Source: CAD feature listing. Evaluate the final solid. Frame: model axes, mm. Give positions to 0.01 mm unless a question says otherwise; leave off trailing zeros. Order: outer loops, then holes, each group sorted by start corner. A loop starts at its lowest first (then second) coordinate and runs counter-clockwise, first axis right, second up. Notation, with made-up numbers: (-8.5, 55.25) - (9.5, 55.25) arc R18 cw to (9.5, 78.25) - close; hole circle Ø7 at (66.5, -14). An arc over 180 degrees is marked (long way). Answer as CSV lines item,"result".
```python
from build123d import *

# Parameters (mm, degrees)
SKETCH1_W           = 62
SKETCH1_H           = 35
BOSS_EXTRUDE1_DEPTH = 5
SKETCH2_R           = 2.5
CUT_EXTRUDE1_DEPTH  = 6
SKETCH3_R           = 2.5
SKETCH3_R_2         = 5
CUT_EXTRUDE2_DEPTH  = 6


with BuildPart() as part:
    # Sketch1 → Boss-Extrude1 (new body)
    with BuildSketch(Plane(origin=(0, 0, 0), x_dir=(1, 0, 0), z_dir=(0, 1, 0))):
        with Locations((31, 17.5)):
            Rectangle(SKETCH1_W, SKETCH1_H)
    extrude(amount=BOSS_EXTRUDE1_DEPTH)

    # Sketch2 → Cut-Extrude1 (cut, through all)
    with BuildSketch(Plane(origin=(0, 5, 0), x_dir=(1, 0, 0), z_dir=(0, 1, 0))):
        with Locations((5, 30)):
            Circle(SKETCH2_R)
        with Locations((5, 5)):
            Circle(SKETCH2_R)
    extrude(amount=-CUT_EXTRUDE1_DEPTH, mode=Mode.SUBTRACT)

    # Sketch3 → Cut-Extrude2 (cut, through all)
    with BuildSketch(Plane(origin=(0, 5, 0), x_dir=(1, 0, 0), z_dir=(0, 1, 0))):
        with Locations((56, 29)):
            Circle(SKETCH3_R)
        with Locations((56, 6)):
            Circle(SKETCH3_R)
        with Locations((33, 28.877597721)):
            Circle(SKETCH3_R)
        with Locations((33, 6)):
            Circle(SKETCH3_R)
        with Locations((44.5, 17.5)):
            Circle(SKETCH3_R_2)
    extrude(amount=-CUT_EXTRUDE2_DEPTH, mode=Mode.SUBTRACT)


solid = part.part
```
(1) Contact query for a flat-ended pin moving along its axis: pin 1 (4.5 mm diameter, centred on x = 56, z = -6, fed in from +Y). Output: stop coordinate, or through.
Completed:
pin 1,"through"
(2) Ray query, line 1 (Z direction, x = 33, y = 2.85); line 2 (Z direction, x = 5, y = 1.7); line 3 (X direction, y = 3.2, z = -28). Return the intervals inside material, ascending. Write a range as from..to.
Completed:
line 1,"-35..-31.38, -26.38..-8.5, -3.5..0"
line 2,"-35..-32.5, -27.5..-7.5, -2.5..0"
line 3,"0..3.5, 6.5..30.66, 35.34..53.71, 58.29..62"
(3) Cut plane C-C (x = 5). Return loops of the section in (y, z).
Completed:
outline,"(0, -35) - (5, -35) - (5, -32.5) - (0, -32.5) - close; (0, -27.5) - (5, -27.5) - (5, -7.5) - (0, -7.5) - close; (0, -2.5) - (5, -2.5) - (5, 0) - (0, 0) - close"
(4) Cut plane A-A (z = -21.5). Return loops of the section in (x, y).
Completed:
outline,"(0, 0) - (41.5, 0) - (41.5, 5) - (0, 5) - close; (47.5, 0) - (62, 0) - (62, 5) - (47.5, 5) - close"
(5) Cut plane D-D (z = -6). Return loops of the section in (x, y), then the cut area to 3 significant figures.
Completed:
outline,"(0, 0) - (2.71, 0) - (2.71, 5) - (0, 5) - close; (7.29, 0) - (30.5, 0) - (30.5, 5) - (7.29, 5) - close; (35.5, 0) - (53.5, 0) - (53.5, 5) - (35.5, 5) - close; (58.5, 0) - (62, 0) - (62, 5) - (58.5, 5) - close"
area,"237 mm²"
(6) Mould query, pull axis Z, two halves, no side actions, for faces 1 (the cylindrical face through (7.385, 2.535, -5.751)), 2 (the flat face through (31, 2, 0)), 3 (the flat face through (31, 0, -18)). Classes: released by +Z, released by -Z, zero draft, split by the parting line, or undercut.
Completed:
face 1,"undercut"
face 2,"released by +Z"
face 3,"zero draft"
(7) Cut plane B-B (x = 44.5). Return loops of the section in (y, z).
Completed:
outline,"(0, -35) - (5, -35) - (5, -22.5) - (0, -22.5) - close; (0, -12.5) - (5, -12.5) - (5, 0) - (0, 0) - close"
